The figure shows three views and two pictorial views of one solid part (mm, origin at its lowest corner). Answer the questions. A direction names the side the tool comes from. Round coordinates to 2 decimals unless told otherwise and drop trailing zeros. Loops run counter-clockwise (first coordinate to the right, second up) from the corner with the lowest first, then second, coordinate; pieces in that order, holes last. Notation, with made-up numbers: (15.25, 12) -> (28.25, 12) arc R13 ccw to (28.25, 36) -> close; hole circle Ø5 at (-25, 60.25). An arc over 180 degrees is marked (long way). Use a Markdown table: item, result. Add a question column.
Q1. Section A-A on x = 14 is taken. Give the vertices of the cut face in (y, z), then the cut area to 3 significant figures.
Q2. Given pin 1 Ø5 at (y, z) = (13.5, 29.5) entering from +X; pin 2 Ø1 at (x, z) = (7.5, 18) entering from -Y; pin 3 Ø6 at (x, z) = (5.5, 20.5) entering from -Y, each flat-ended and moving along its own axis, determine where each tip first touches the part or whether it passes through.
Q3. Which of the six approach directions +Z, -Z, +X, -X, +Y, -Y give full straight-line access (tool end or side, diameter ignored) to the marked faces 1, 2 and 3?
Q4. Consider line 1 (Z direction, x = 9, y = 2); line 2 (X direction, y = 15.25, z = 25); line 3 (Y direction, x = 9.75, z = 16.5). Determine where each line is inside the solid, lowest interval first.
Q5. Section C-C on z = 28 is taken. Give the vertices of the cut face in (x, y), then the cut area to 3 significant figures.
Q6. Section D-D on z = 14.5 is taken. Give the vertices of the cut face in (x, y), then the cut area to 3 significant figures.
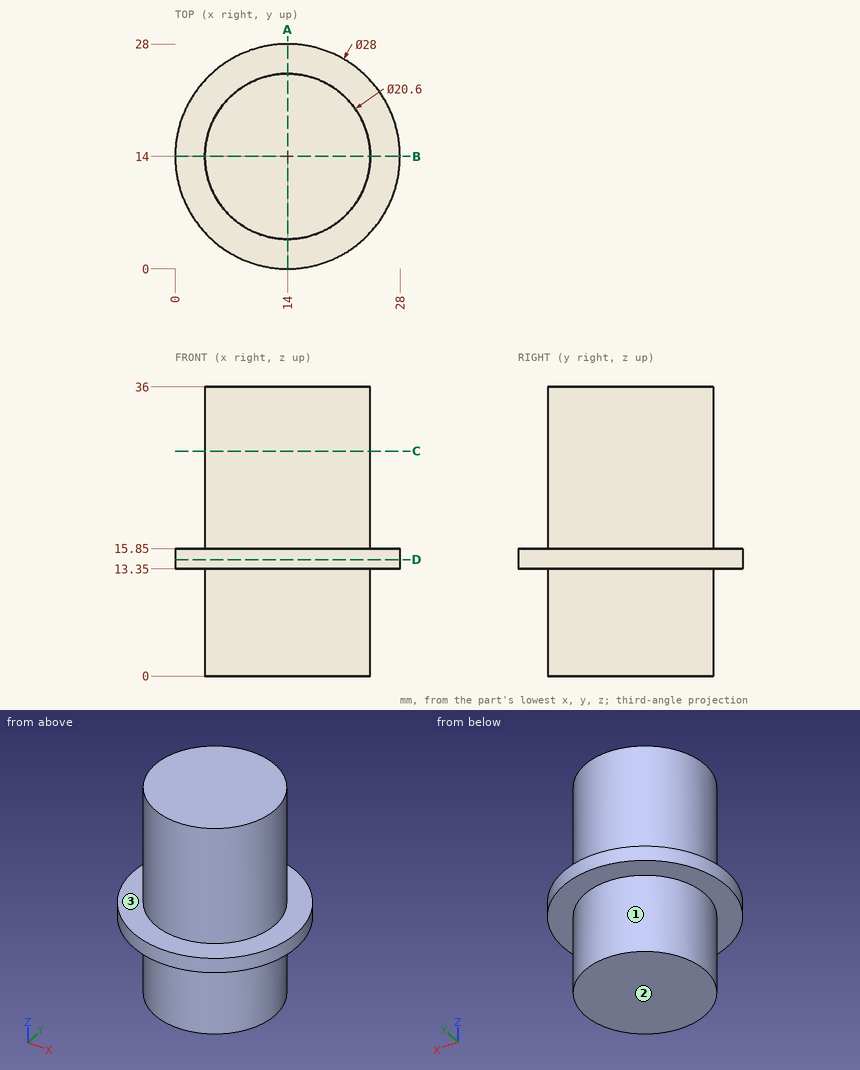
Checked values:
| question | item | result |
|---|---|---|
| 1 | outline | (0, 13.35) -> (3.7, 13.35) -> (3.7, 0) -> (24.3, 0) -> (24.3, 13.35) -> (28, 13.35) -> (28, 15.85) -> (24.3, 15.85) -> (24.3, 36) -> (3.7, 36) -> (3.7, 15.85) -> (0, 15.85) -> close |
| 1 | area | 760 mm2 |
| 2 | pin 1 | stops at x = 24.3 |
| 2 | pin 2 | stops at y = 5.63 |
| 2 | pin 3 | stops at y = 5.29 |
| 3 | face 1 | -Z |
| 3 | face 2 | -Z, +X, -X, +Y, -Y |
| 3 | face 3 | +Z |
| 4 | line 1 | z = 13.35 to 15.85 |
| 4 | line 2 | x = 3.78 to 24.22 |
| 4 | line 3 | y = 4.62 to 23.38 |
| 5 | outline | circle Ø20.6 at (14, 14) |
| 5 | area | 333 mm2 |
| 6 | outline | circle Ø28 at (14, 14) |
| 6 | area | 616 mm2 |
